```python
from build123d import *

# Parameters (mm, degrees)
BOSS_EXTRUDE1_DEPTH = 4.7625
SKETCH3_R           = 1.25
CUT_EXTRUDE1_DEPTH  = 266.210067011
SKETCH4_R           = 1.75
CUT_EXTRUDE2_DEPTH  = 266.210067011


with BuildPart() as part:
    # Sketch1 → Boss-Extrude1 (new body)
    with BuildSketch(Plane.XY):
        with BuildLine():
            Line((0, 12.64261775), (-254, 12.64261775))
            Line((-254, 12.64261775), (-254, -12.64261775))
            Line((-254, -12.64261775), (-254, -76.14261775))
            Line((-254, -76.14261775), (-247.65, -76.14261775))
            Line((-247.65, -76.14261775), (-247.65, -12.64261775))
            Line((-247.65, -12.64261775), (0, -12.64261775))
            ThreePointArc((0, -12.64261775), (12.64261775, 0), (0, 12.64261775))
        make_face()
    extrude(amount=BOSS_EXTRUDE1_DEPTH)

    # Sketch3 → Cut-Extrude1 (cut, through all)
    with BuildSketch(Plane.XY.offset(4.7625)):
        with Locations((-15, 0)):
            Circle(SKETCH3_R)
        with Locations((-20, 0)):
            Circle(SKETCH3_R)
    extrude(amount=-CUT_EXTRUDE1_DEPTH, mode=Mode.SUBTRACT)

    # Sketch4 → Cut-Extrude2 (cut, through all)
    with BuildSketch(Plane.XY.offset(4.7625)):
        Circle(SKETCH4_R)
    extrude(amount=-CUT_EXTRUDE2_DEPTH, mode=Mode.SUBTRACT)


solid = part.part
```
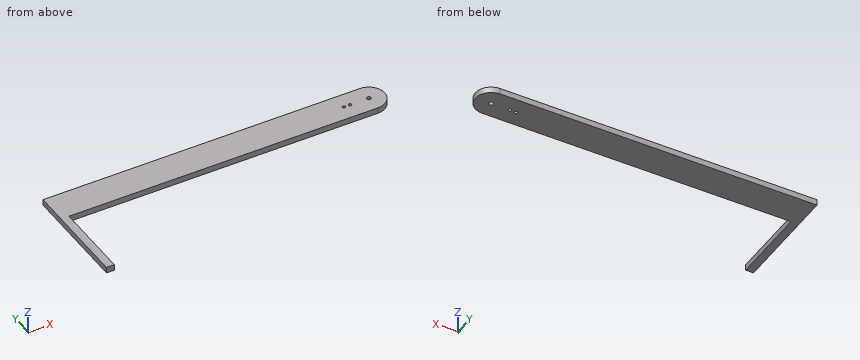
Model file for the job. Use its own axes, mm. Coordinates: 2 decimals unless noted, no trailing zeros. Loops run counter-clockwise (first coordinate to the right, second up) from the corner with the lowest first, then second, coordinate; pieces in that order, holes last. Notation, with made-up numbers: (53, 7) - (93, 7) arc R15 ccw to (93, 23) - close; hole circle Ø3 at (-5.75, 0). An arc over 180 degrees is marked (long way). Write item = value, one per line. Start each with the question number.
Item 1: Saw through at A-A, the plane z = 3.4. List the corners of the cut face in (x, y), then the cut area to 3 significant figures.
Item 2: Saw through at C-C, the plane y = -41. List the corners of the cut face in (x, z), then the cut area to 3 significant figures.
Item 3: Saw through at B-B, the plane x = -25. List the corners of the cut face in (y, z), then the cut area to 3 significant figures.
Item 4: Wall check: probe 1 along Y at (x, z) = (-20, 2.4); probe 2 along X at (y, z) = (-28, 4.4); probe 3 along Y at (x, z) = (-166.5, 1.25). Give the ranges that are in metal, low to high. Write a range as [from, to].
Answers:
q1.outline = (-254, -76.14) - (-247.65, -76.14) - (-247.65, -12.64) - (0, -12.64) arc R12.64 ccw to (0, 12.64) - (-254, 12.64) - close; hole circle Ø2.5 at (-20, 0); hole circle Ø2.5 at (-15, 0); hole circle Ø3.5 at (0, 0)
q1.area = 7,060 mm2
q2.outline = (-254, 0) - (-247.65, 0) - (-247.65, 4.76) - (-254, 4.76) - close
q2.area = 30.2 mm2
q3.outline = (-12.64, 0) - (12.64, 0) - (12.64, 4.76) - (-12.64, 4.76) - close
q3.area = 120 mm2
q4.probe_1 = [-12.64, -1.25], [1.25, 12.64]
q4.probe_2 = [-254, -247.65]
q4.probe_3 = [-12.64, 12.64]
